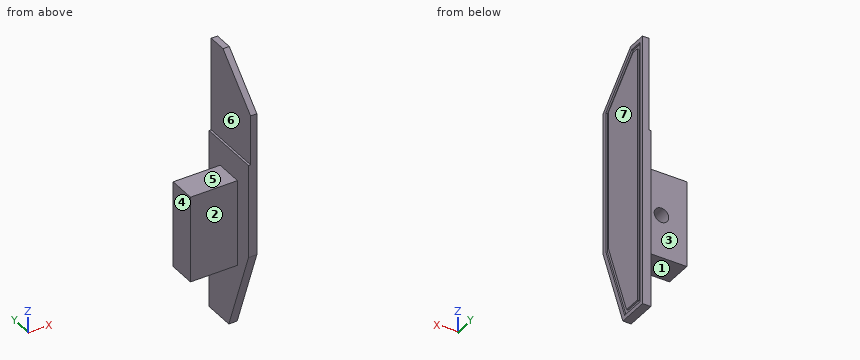
Autodesk Inventor part; units mm, degrees
ref_plane "YZ Plane" through (0, 0, 0) normal (1, 0, 0) x (0, 1, 0)
ref_plane "XZ Plane" through (0, 0, 0) normal (0, 1, 0) x (-1, 0, 0)
ref_plane "XY Plane" through (0, 0, 0) normal (0, 0, 1) x (1, 0, 0)
sketch "Эскиз1" plane through (0, 0, 0) normal (1, 0, 0) x (0, 1, 0)
  line L0 (-7.5, -32.85) -> (7.5, -32.85)
  line L1 (7.5, -32.85) -> (7.5, 32.85)
  line L2 (7.5, 32.85) -> (-7.5, 32.85)
  line L3 (-7.5, 32.85) -> (-7.5, -32.85)
  line L4 (-7.5, -32.85) -> (7.5, 32.85) construction
  line L5 (7.5, -32.85) -> (-7.5, 32.85) construction
  line L6 (0, -32.85) -> (0, -16.55) construction
  line L7 (3.3, 4.25) -> (-3.3, 4.25)
  line L8 (-3.3, 4.25) -> (-3.3, -16.55)
  line L9 (-3.3, -16.55) -> (3.3, -16.55)
  line L10 (3.3, -16.55) -> (3.3, 4.25)
  line L11 (7.5, 32.85) -> (-7.5, 32.85)
  line L12 (-7.5, 32.85) -> (-7.5, 10.35)
  line L13 (-7.5, 10.35) -> (7.5, 10.35)
  line L14 (7.5, 10.35) -> (7.5, 32.85)
  line L15 (0, -32.85) -> (-7.5, -12.2439)
  line L16 (0, -32.85) -> (21.9285, -32.85) construction
  point P0 (0, 0)
  point P1 (7.5, 10.35)
  dimension "d0" = 15
  dimension "d1" = 65.7
  dimension "d2" = 16.3
  dimension "d3" = 6.6
  dimension "d4" = 20.8
  dimension "d5" = 22.5
  dimension "d25" = 110
extrude "Выдавливание1" add sketch "Эскиз1" along normal blind 2 contours L15 L3 L13 L1 L0 | L3 L2 L1 L13 | L10 L9 L8 L7
extrude "Выдавливание2" add sketch "Эскиз1" against normal blind 11.3 contours L10 L9 L8 L7
extrude "Выдавливание3" cut sketch "Эскиз1" along normal blind 0.5 contours L3 L2 L1 L13
chamfer "Фаска2" distance 10.5 angle 45 1 edges at (1.25, -7.5, 32.85)
sketch "Эскиз2" plane through (2, 0, 0) normal (1, 0, 0) x (0, 0, -1)
  line L0 (-22.35, -7.5) -> (-32.85, 3)
  line L1 (-22.35, -7.5) -> (12.2439, -7.5)
  line L2 (32.85, 0) -> (32.85, 7.5)
  line L3 (32.85, 7.5) -> (-32.85, 7.5)
  line L4 (-32.85, 7.5) -> (-32.85, 3)
  line L5 (12.2439, -7.5) -> (32.85, 0)
  line L6 (31.85, 0.7002) -> (12.0676, -6.5)
  line L7 (12.0676, -6.5) -> (-21.9358, -6.5)
  line L8 (-21.9358, -6.5) -> (-31.85, 3.4142)
  line L9 (-31.85, 3.4142) -> (-31.85, 6.5)
  line L10 (-31.85, 6.5) -> (31.85, 6.5)
  line L11 (31.85, 6.5) -> (31.85, 0.7002)
  line L12 (30.85, 5.5) -> (-30.85, 5.5)
  line L13 (-30.85, 5.5) -> (-30.85, 3.8284)
  line L14 (-30.85, 3.8284) -> (-21.5216, -5.5)
  line L15 (-21.5216, -5.5) -> (11.8913, -5.5)
  line L16 (11.8913, -5.5) -> (30.85, 1.4004)
  line L17 (30.85, 1.4004) -> (30.85, 5.5)
  point P0 (0, 0)
  dimension "d26" = 1
  dimension "d32" = 1
extrude "Выдавливание5" cut sketch "Эскиз2" against normal blind 0.4 contours L6 L7 L8 L9 L10 L11
sketch "Эскиз3" plane through (-11.3, 3.3, -16.55) normal (0, 1, 0) x (1, 0, 0)
  line L0 (0, 0) -> (0, -20.8)
  line L1 (0, 0) -> (6.1, 0) construction
  line L2 (6.1, 0) -> (6.1, -10.4) construction
  line L3 (6.1, -10.4) -> (0, -10.4) construction
  line L4 (0, -10.4) -> (0, 0) construction
  circle A0 centre (6.1, -10.4) radius 1.75
  point P0 (11.3, -16.55)
  dimension "d27" = 6.1
  dimension "d28" = 10.4
  dimension "d29" = 3.5
extrude "Выдавливание6" cut sketch "Эскиз3" against normal blind 5
properties part number "switch_cap_bl"
Verification items for the finished model (mm, model axes). Face numbers are marked on the shaded views. A direction names the side the tool comes from. Give positions to 0.01 mm unless a question says otherwise; leave off trailing zeros. Write each loop counter-clockwise with the first axis right and the second up, starting at its lowest first coordinate (ties: lowest second). Pieces come first, ordered by that corner, then holes. Notation, with made-up numbers: M 60.5,86 L 68.5,86 A23 cw 68.5,111 Z; hole C 85.25,-33 d6. An arc over 180 degrees is marked long. Put each result on its own line as item: value. Start each with the question number.
1. Section check C-C (y = -4.25). Record the cut outline in (x, z), and give its area (3 significant figures).
2. Scan lines: line 1 along Z through (x, y) = (-5.2, 1.25); line 2 along X through (y, z) = (1.05, -6.15); line 3 along X through (y, z) = (-5.25, -3.5). Record each from-to range of solid material in increasing order. Write a range as [from, to].
3. Set-up check for the marked faces 1, 2, 3 and 4: record each of +Z, -Z, +X, -X, +Y, -Y from which the full face is reachable in a straight line by a thin tool's end or side.
4. Go/stop test with flat-tipped pins: pin 1 Ø4 at (x, z) = (-6, -14) entering from +Y; pin 2 Ø2 at (x, z) = (-5.2, -6.15) entering from -Y; pin 3 Ø2 at (x, y) = (-7.5, 1.5) entering from -Z; pin 4 Ø6 at (x, z) = (-4, 11) entering from +Y. Record where each tip stops, or that it passes through.
5. Section check A-A (z = -6.15). Record the cut outline in (x, y).
6. Section check D-D (z = 17.5). Record the cut outline in (x, y).
7. Draft check along X on the marked faces 5, 6 and 7. Enter one of: +X half, -X half, draft (parallel to the pull), parting line (faces both ways), or undercut.
8. Section check B-B (x = -5.2). Record the cut outline in (y, z).
Answer list:
1. outline: M 0,-21.17 L 2,-21.17 L 2,-18.25 L 1.6,-18.25 L 1.6,-15.33 L 2,-15.33 L 2,22.77 L 1.6,22.77 L 1.6,24.19 L 2,24.19 L 2,25.6 L 0.5,25.6 L 0.5,10.35 L 0,10.35 Z
1. area: 84.2 mm2
2. line 1: [-16.55, -7.9], [-4.4, 4.25]
2. line 2: [-11.3, -6.95], [-3.45, 2]
2. line 3: [0, 2]
3. face 1: -Z, -X, +Y, -Y
3. face 2: +Z, -Z, -X, -Y
3. face 3: +Z, -Z, -X, +Y
3. face 4: +Z, -Z, -X, +Y, -Y
4. pin 1: y = 3.3
4. pin 2: y = -3.3
4. pin 3: z = -16.55
4. pin 4: through
5. outline: M -11.3,-3.3 L 0,-3.3 L 0,-7.5 L 2,-7.5 L 2,-6.5 L 1.6,-6.5 L 1.6,-5.5 L 2,-5.5 L 2,5.5 L 1.6,5.5 L 1.6,6.5 L 2,6.5 L 2,7.5 L 0,7.5 L 0,3.3 L -3.45,3.3 L -3.45,-1.7 L -6.95,-1.7 L -6.95,3.3 L -11.3,3.3 Z
6. outline: M 0.5,-7.5 L 2,-7.5 L 2,-6.5 L 1.6,-6.5 L 1.6,-5.5 L 2,-5.5 L 2,5.5 L 1.6,5.5 L 1.6,6.5 L 2,6.5 L 2,7.5 L 0.5,7.5 Z
7. face 5: draft
7. face 6: -X half
7. face 7: +X half
8. outline: M -3.3,-16.55 L 3.3,-16.55 L 3.3,-7.9 L -1.7,-7.9 L -1.7,-4.4 L 3.3,-4.4 L 3.3,4.25 L -3.3,4.25 Z
